from build123d import *

# Parameters (mm, degrees)
F0_W     = 1524
F0_H     = 508
F1_DEPTH = 381
F2_W     = 1270
F2_H     = 381
F3_DEPTH = 254
F5_DEPTH = 1270
F6_W     = 1524
F6_H     = 508
F7_DEPTH = 25.4


with BuildPart() as f1:
    # F0 (on Top) → F1 (new body)
    with BuildSketch(Plane.XY):
        Rectangle(F0_W, F0_H)
    extrude(amount=F1_DEPTH)

    # F2 (on face) → F3 (cut)
    with BuildSketch(Plane(origin=(0, 0, 0), x_dir=(1, 0, 0), z_dir=(0, 0, -1))):
        Rectangle(F2_W, F2_H)
    extrude(amount=-F3_DEPTH, mode=Mode.SUBTRACT)

    # F4 (on face) → F5 (join, through all)
    with BuildSketch(Plane(origin=(635, 0, 0), x_dir=(0, -1, 0), z_dir=(-1, 0, 0))):
        with BuildLine():
            Line((-101.6, 254), (-190.5, 254))
            Line((-190.5, 254), (-190.5, 165.1))
            ThreePointArc((-190.5, 165.1), (-146.05, 209.55), (-101.6, 165.1))
            Line((-101.6, 165.1), (-101.6, 254))
        make_face()
    extrude(amount=F5_DEPTH)

    # F6 (on face) → F7 (join)
    with BuildSketch(Plane.XY.offset(381)):
        Rectangle(F6_W, F6_H)
    extrude(amount=F7_DEPTH)


solid = f1.part
CAD build for the part. Positions are in the model's coordinates, mm. A direction names the side the tool comes from. Give positions to 0.01 mm unless a question says otherwise; leave off trailing zeros. Loops run counter-clockwise (first coordinate to the right, second up) from the corner with the lowest first, then second, coordinate; pieces in that order, holes last. Notation, with made-up numbers: M 19,-33 L 65,-33 A29 cw 65,5 Z; hole C 18.5,-6.75 d2. An arc over 180 degrees is marked long. Answer in a Markdown table with one row per item. Add a question column.
Item 1: Band-saw the part on C-C on x = 376. Give the cut face in (y, z), then the cut area to 3 significant figures.
Item 2: Tool access for faces 4 (the face through (-11, -222, 0)), 5 (the face through (-9, -46, 254)): list every direction of +Z, -Z, +X, -X, +Y, -Y with a clear straight run to the whole face (end or side of a thin tool).
Item 3: Drop flat-ended pins along their axis: P1, Ø3, axis at x = -475, y = 118.5, coming from the -Z side; P2, Ø4, axis at x = -111.5, y = -23.5, coming from the -Z side. Give the stop position or say it passes through.
Item 4: Band-saw the part on A-A on z = 121. Give the cut face in (x, y), then the cut area to 3 significant figures.
Item 5: Probe probe 1 along X at (y, z) = (-93, 219); probe 2 along Y at (x, z) = (-515.5, 99); probe 3 along Y at (x, z) = (63, 185.5). List the from-to ranges inside material, lowest first.
Item 6: Band-saw the part on B-B on y = 146.05. Give the cut face in (x, z), then the cut area to 3 significant figures.
Item 7: Band-saw the part on D-D on y = -5. Give the cut face in (x, z).
Item 8: Mould opens along X. For faces 1 (the face through (-11, 4, 406.4)), 2 (the face through (762, -4, 200)), 3 (the face through (9, 101.6, 209)) say: +X half, -X half, draft (parallel to the pull), parting line (faces both ways), or undercut.
Reply:
| question | item | result |
|---|---|---|
| 1 | outline | M -254,0 L -190.5,0 L -190.5,254 L 101.6,254 L 101.6,165.1 A44.45 cw 190.5,165.1 L 190.5,0 L 254,0 L 254,406.4 L -254,406.4 Z |
| 1 | area | 114,000 mm^2 |
| 2 | face 4 | -Z, +X, -X, +Y, -Y |
| 2 | face 5 | -Z |
| 3 | P1 | stops at z = 198.74 |
| 3 | P2 | stops at z = 254 |
| 4 | outline | M -762,-254 L 762,-254 L 762,254 L -762,254 Z; hole M -635,-190.5 L 635,-190.5 L 635,190.5 L -635,190.5 Z |
| 4 | area | 290,000 mm^2 |
| 5 | probe 1 | x = -762 to -635, 635 to 762 |
| 5 | probe 2 | y = -254 to -190.5, 190.5 to 254 |
| 5 | probe 3 | y = -254 to -190.5, 101.6 to 106.56, 185.54 to 254 |
| 6 | outline | M -762,0 L -635,0 L -635,209.55 L 635,209.55 L 635,0 L 762,0 L 762,406.4 L -762,406.4 Z |
| 6 | area | 353,000 mm^2 |
| 7 | outline | M -762,0 L -635,0 L -635,254 L 635,254 L 635,0 L 762,0 L 762,406.4 L -762,406.4 Z |
| 8 | face 1 | draft |
| 8 | face 2 | +X half |
| 8 | face 3 | undercut |
